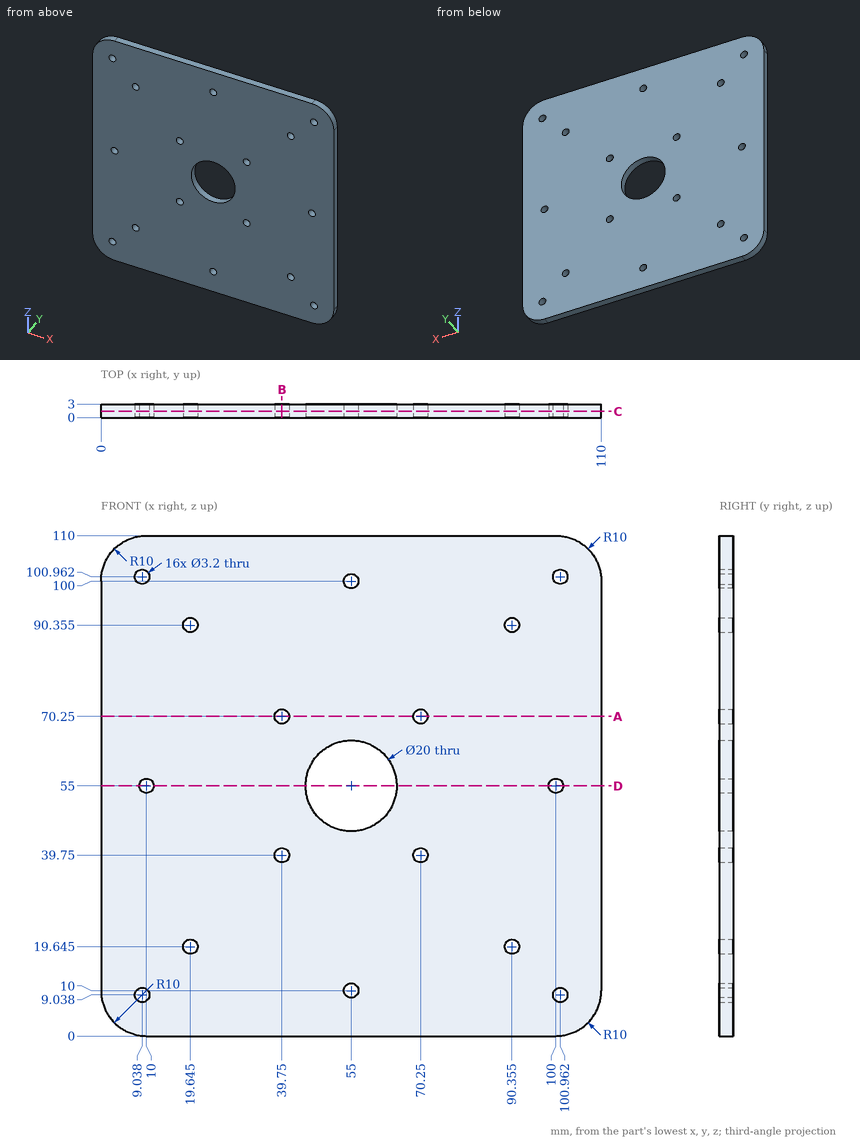
Answer from the drawing. Dimensions are ordinates in mm from the lowest x, y and z of the part. Round coordinates to 2 decimals unless told otherwise and drop trailing zeros. Write each loop counter-clockwise with the first axis right and the second up, starting at its lowest first coordinate (ties: lowest second). Pieces come first, ordered by that corner, then holes. Notation, with made-up numbers: (43.5, 6.25) - (89.5, 6.25) arc R28 cw to (89.5, 34.25) - close; hole circle Ø2 at (34, 41.5). An arc over 180 degrees is marked (long way). One line per item, written item: value.
Q1. Find section D-D (z = 55). Determine the outline of the cut face in (x, y), and give its area (3 significant figures).
The answers:
outline: (0, 0) - (8.4, 0) - (8.4, 3) - (0, 3) - close; (11.6, 0) - (45, 0) - (45, 3) - (11.6, 3) - close; (65, 0) - (98.4, 0) - (98.4, 3) - (65, 3) - close; (101.6, 0) - (110, 0) - (110, 3) - (101.6, 3) - close
area: 251 mm2
Q2. Find section B-B (x = 39.75). Determine the outline of the cut face in (y, z).
The answers:
outline: (0, 0) - (3, 0) - (3, 38.15) - (0, 38.15) - close; (0, 41.35) - (3, 41.35) - (3, 68.65) - (0, 68.65) - close; (0, 71.85) - (3, 71.85) - (3, 110) - (0, 110) - close
Q3. Find section A-A (z = 70.25). Determine the outline of the cut face in (x, y), and give its area (3 significant figures).
The answers:
outline: (0, 0) - (38.15, 0) - (38.15, 3) - (0, 3) - close; (41.35, 0) - (68.65, 0) - (68.65, 3) - (41.35, 3) - close; (71.85, 0) - (110, 0) - (110, 3) - (71.85, 3) - close
area: 311 mm2
Q4. Straight lines are drawn through the part: line 1 (Z direction, x = 70, y = 1.5); line 2 (X direction, y = 1.65, z = 70.25); line 3 (X direction, y = 1.5, z = 89.5). For each, find the intervals that lie inside material, in ascending order. Write a range as from..to.
The answers:
line 1: z = 0..38.17, 41.33..68.67, 71.83..110
line 2: x = 0..38.15, 41.35..68.65, 71.85..110
line 3: x = 0..18.29, 21..89, 91.71..110
Q5. Find section C-C (y = 1.4). Count the separate pieces of the cut face and the enclosed holes in it, and give its area (3 significant figures).
The answers:
separate pieces: 1
enclosed holes: 17
area: 11,600 mm2
